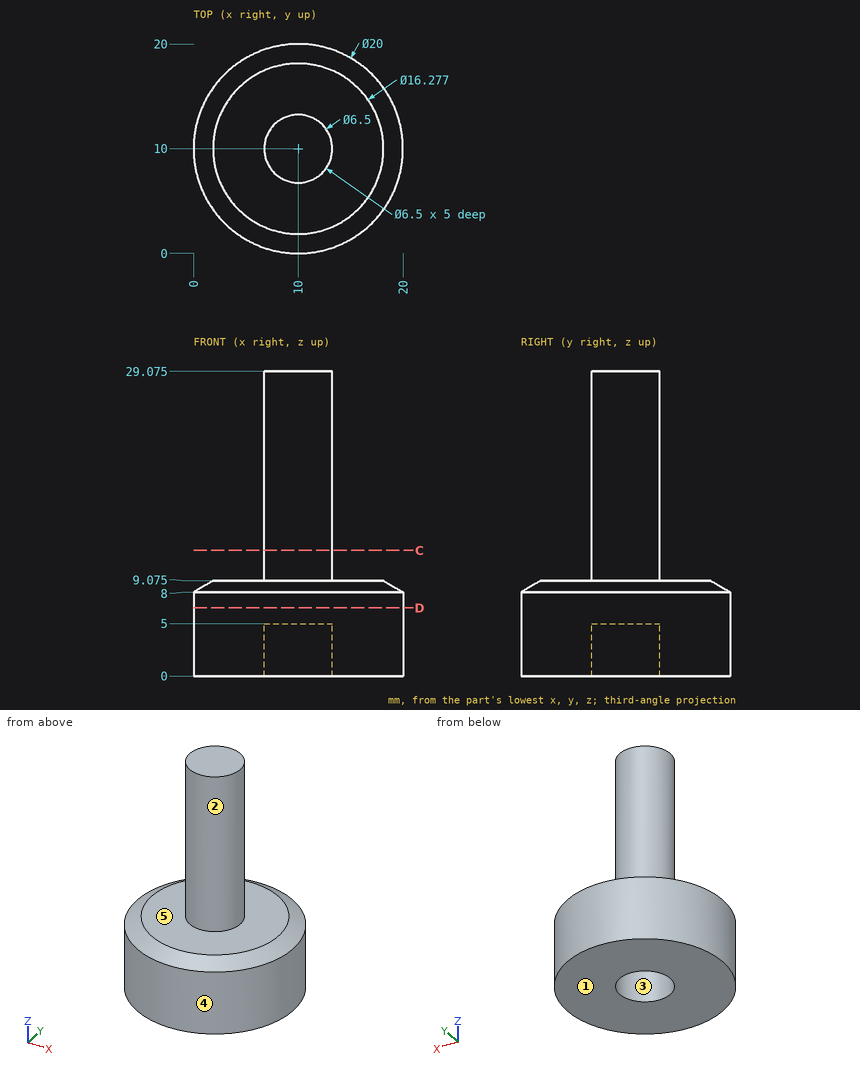
The drawing under review shows one solid part. Ordinate dimensions are in mm from its lowest x, y, z. A direction names the side the tool comes from. Coordinates: 2 decimals unless noted, no trailing zeros. Loops run counter-clockwise (first coordinate to the right, second up) from the corner with the lowest first, then second, coordinate; pieces in that order, holes last. Notation, with made-up numbers: M 69.5,64.25 L 85.5,64.25 A21 ccw 85.5,69.25 Z; hole C 60.5,56.25 d11. An arc over 180 degrees is marked long. Use one line per item in the form item = value.
(1) Clearance check with flat-ended pins moving along their axes: P1, Ø2, axis at y = 8, z = 15.5, coming from the -X side; P2, Ø8, axis at x = 5, z = 16.5, coming from the -Y side; P3, Ø6, axis at y = 15, z = 23, coming from the -X side; P4, Ø1, axis at y = 5.5, z = 24.5, coming from the +X side. State where each tip first meets the part, or that it passes through.
Return value:
P1 = 6.91
P2 = 6.91
P3 = 7.44
P4 = through
(2) For the marked faces 4 and 5, list the 3-axis set-ups (+Z, -Z, +X, -X, +Y, -Y) from which the entire face can be reached by the end or side of a thin tool; tool diameter is ignored.
Return value:
face_4 = +Z, -Z
face_5 = +Z
(3) Consider section D-D (z = 6.5). Write out the cut boundary in (x, y), and give its area (3 significant figures).
Return value:
outline = C 10,10 d20
area = 314 mm2
(4) Consider section C-C (z = 12). Write out the cut boundary in (x, y), and give its area (3 significant figures).
Return value:
outline = C 10,10 d6.5
area = 33.2 mm2
(5) Draft analysis for pull direction X (two halves, no side actions). For the marked faces 1, 2 and 3, state which applies: pulls with the +X half, pulls with the -X half, needs draft (parallel to the pull), parting line crosses it, or undercut.
Return value:
face_1 = needs draft
face_2 = parting line crosses it
face_3 = undercut
(6) For line 1 along Y through (x, z) = (10, 2); line 2 along Z through (x, y) = (15.75, 9.5) (1 decimal), list the stretches that pass through material, from the lowest coordinate up. Write a range as from..to.
Return value:
line_1 = 0..6.75, 13.25..20
line_2 = 0..9.1
